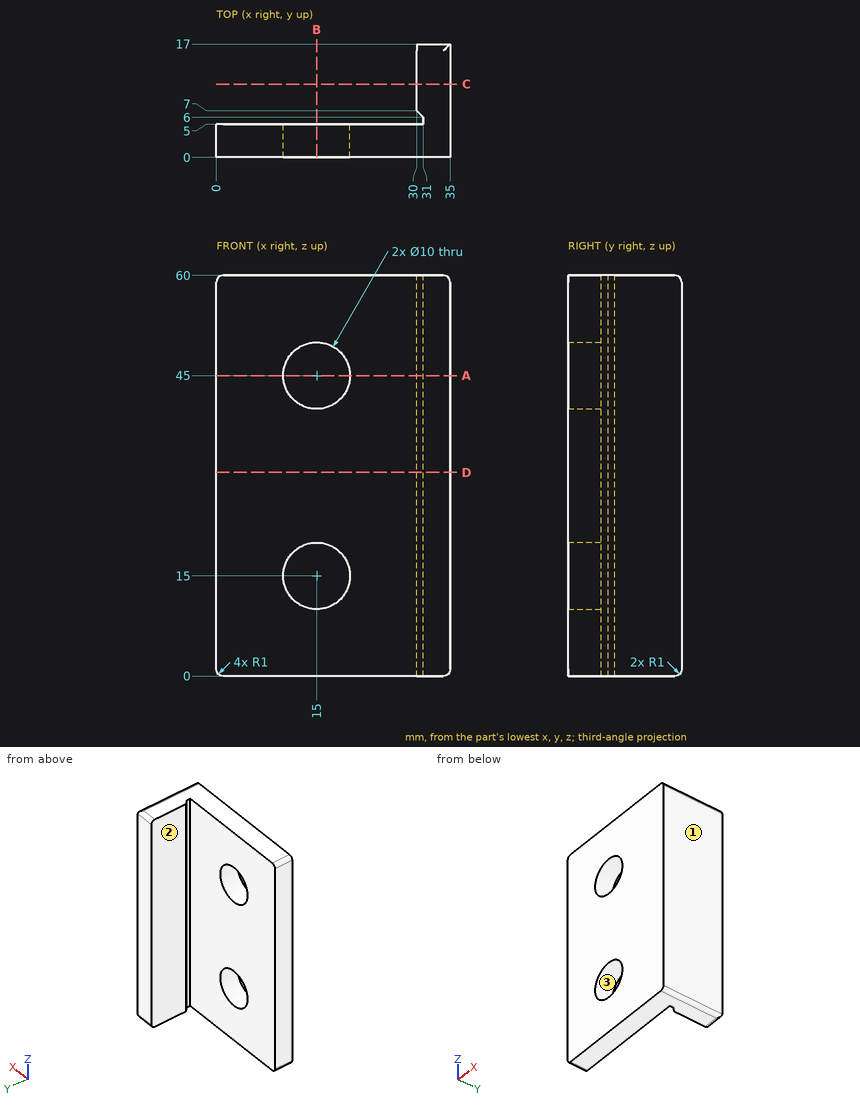
Could you check a few things on this drawing? It's one solid part, dimensions in mm from its lowest x, y, z. Coordinates: 2 decimals unless noted, no trailing zeros. Write each loop counter-clockwise with the first axis right and the second up, starting at its lowest first coordinate (ties: lowest second). Pieces come first, ordered by that corner, then holes.
1) Thinking about a two-plate mould opening in X: for the marked faces 1, 2 and 3, which applies, +X half, -X half, draft (parallel to the pull), parting line (faces both ways), or undercut?
Filled in:
face 1: +X half
face 2: -X half
face 3: undercut
2) If I drill on line 1 (Z direction, x = 15, y = 1.35); line 2 (X direction, y = 3.35, z = 45); line 3 (Z direction, x = 11, y = 3.25), over which ranges is the centre line in solid material (lowest first)?
Filled in:
line 1: z = 0 to 10, 20 to 40, 50 to 60
line 2: x = 0 to 10, 20 to 35
line 3: z = 0 to 12, 18 to 42, 48 to 60
3) If we section it at A-A (z = 45): List the corners of the cut face in (x, y) for me, plus the area to 4 significant figures.
Filled in:
outline: (0, 0) - (10, 0) - (10, 5) - (0, 5) - close; (20, 0) - (35, 0) - (35, 17) - (30, 17) - (30, 7) - (31, 6) - (31, 5) - (20, 5) - close
area: 183.5 mm2
4) If we section it at C-C (y = 11): List the corners of the cut face in (x, z) for me.
Filled in:
outline: (30, 0) - (34, 0) arc R1 ccw to (35, 1) - (35, 59) arc R1 ccw to (34, 60) - (30, 60) - close
5) If we section it at B-B (x = 15): List the corners of the cut face in (y, z) for me.
Filled in:
outline: (0, 0) - (5, 0) - (5, 10) - (0, 10) - close; (0, 20) - (5, 20) - (5, 40) - (0, 40) - close; (0, 50) - (5, 50) - (5, 60) - (0, 60) - close
6) If we section it at D-D (z = 30.5): List the corners of the cut face in (x, y) for me, plus the area to 4 significant figures.
Filled in:
outline: (0, 0) - (35, 0) - (35, 17) - (30, 17) - (30, 7) - (31, 6) - (31, 5) - (0, 5) - close
area: 233.5 mm2
7) I'm going to push flat-ended pins straight in: pin 1 (3 mm diameter, centred on x = 25.5, z = 12.5, fed in from +Y); pin 2 (1.1 mm diameter, centred on y = 5.5, z = 35.5, fed in from -X); pin 3 (4 mm diameter, centred on y = 10.5, z = 45.5, fed in from -X); pin 4 (8 mm diameter, centred on x = 15, z = 45, fed in from -Y). Where does each tip first touch, or does it pass through?
Filled in:
pin 1: stops at y = 5
pin 2: stops at x = 0
pin 3: stops at x = 30
pin 4: passes through
